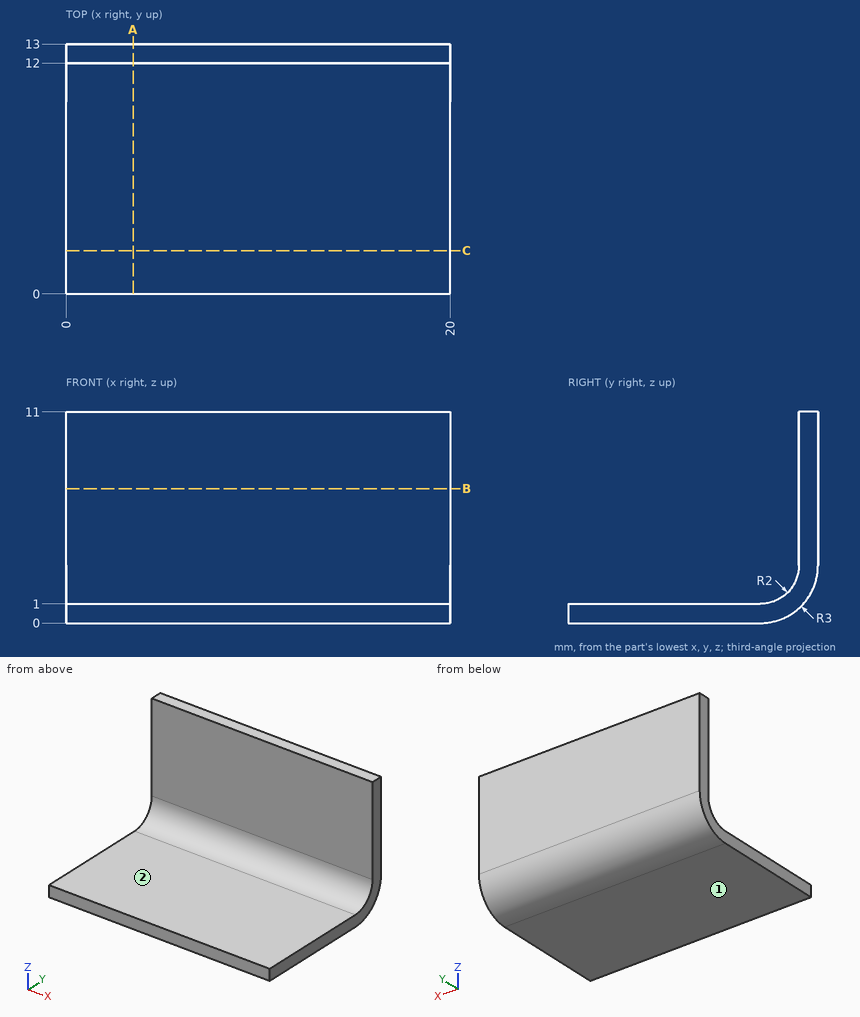
Geometry check sheet. Reference: drawing and pictorial views, mm from the part's lowest x, y, z. A direction names the side the tool comes from. Coordinates: 2 decimals unless noted, no trailing zeros. Order: outer loops, then holes, each group sorted by start corner. A loop starts at its lowest first (then second) coordinate and runs counter-clockwise, first axis right, second up. Notation, with made-up numbers: (-27, 9.5) - (-6, 9.5) arc R22 ccw to (-6, 31.5) - close; hole circle Ø6 at (-22, 17). An arc over 180 degrees is marked (long way). Answer in a Markdown table with one row per item. Add a question column.
1) Cross-section at C-C, the plane y = 2.25. Record the cut outline in (x, z).
2) Gauge pin test, flat ends, axial feed: P1, Ø3, axis at x = 7, y = 3, coming from the +Z side; P2, Ø2.5, axis at x = 14, z = 6.5, coming from the -Y side. Record the tip position at first contact, or that the pin passes through.
3) Cross-section at B-B, the plane z = 7. Record the cut outline in (x, y).
4) Material ranges on line 1 along Y through (x, z) = (5, 7.5); line 2 along Z through (x, y) = (19, 6.75); line 3 along Y through (x, z) = (17.75, 1.25), recorded low to high. Write a range as [from, to].
5) Cross-section at A-A, the plane x = 3.5. Record the cut outline in (y, z).
6) Set-up check for the marked faces 1 and 2: record each of +Z, -Z, +X, -X, +Y, -Y from which the full face is reachable in a straight line by a thin tool's end or side.
Check result:
| question | item | result |
|---|---|---|
| 1 | outline | (0, 0) - (20, 0) - (20, 1) - (0, 1) - close |
| 2 | P1 | stops at z = 1 |
| 2 | P2 | stops at y = 12 |
| 3 | outline | (0, 12) - (20, 12) - (20, 13) - (0, 13) - close |
| 4 | line 1 | y = [12, 13] |
| 4 | line 2 | z = [0, 1] |
| 4 | line 3 | y = [10.97, 12.44] |
| 5 | outline | (0, 0) - (10, 0) arc R3 ccw to (13, 3) - (13, 11) - (12, 11) - (12, 3) arc R2 cw to (10, 1) - (0, 1) - close |
| 6 | face 1 | -Z, +X, -X, +Y, -Y |
| 6 | face 2 | +Z, +X, -X, -Y |
